Job drawing, mm, ordinate dimensions from the low corner. One solid piece. A direction names the side the tool comes from. Give positions to 0.01 mm unless a question says otherwise; leave off trailing zeros. Loops run counter-clockwise (first coordinate to the right, second up) from the corner with the lowest first, then second, coordinate; pieces in that order, holes last. Notation, with made-up numbers: (36, 48) -> (56, 48) arc R27 ccw to (56, 86) -> close; hole circle Ø9 at (7, -11). An arc over 180 degrees is marked (long way). Use one line per item in the form item = value.
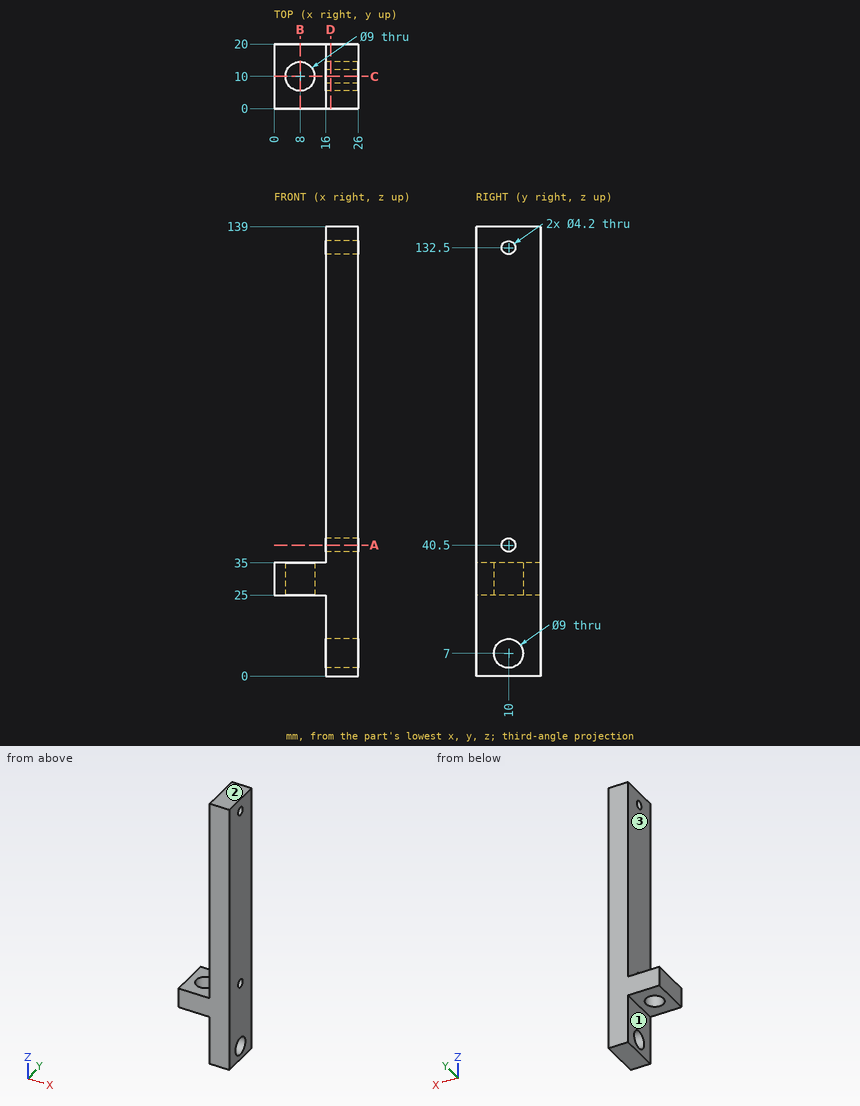
1. Cut at A-A, the plane z = 40.5. Write the cut outline in (x, y), then the cut area to 3 significant figures.
Result sheet:
outline = (16, 0) -> (26, 0) -> (26, 7.9) -> (16, 7.9) -> close; (16, 12.1) -> (26, 12.1) -> (26, 20) -> (16, 20) -> close
area = 158 mm^2
2. Cut at C-C, the plane y = 10. Write the cut outline in (x, z).
Result sheet:
outline = (0, 25) -> (3.5, 25) -> (3.5, 35) -> (0, 35) -> close; (12.5, 25) -> (16, 25) -> (16, 11.5) -> (26, 11.5) -> (26, 38.4) -> (16, 38.4) -> (16, 35) -> (12.5, 35) -> close; (16, 0) -> (26, 0) -> (26, 2.5) -> (16, 2.5) -> close; (16, 42.6) -> (26, 42.6) -> (26, 130.4) -> (16, 130.4) -> close; (16, 134.6) -> (26, 134.6) -> (26, 139) -> (16, 139) -> close
3. Cut at B-B, the plane x = 8. Write the cut outline in (y, z).
Result sheet:
outline = (0, 25) -> (5.5, 25) -> (5.5, 35) -> (0, 35) -> close; (14.5, 25) -> (20, 25) -> (20, 35) -> (14.5, 35) -> close
4. Drill centre lines: line 1 (Z direction, x = 21.25, y = 10); line 2 (Y direction, x = 22.25, z = 132.5); line 3 (Z direction, x = 20.5, y = 9.5). Where is each one in solid material? Low to high.
Result sheet:
line_1 = 0 to 2.5, 11.5 to 38.4, 42.6 to 130.4, 134.6 to 139
line_2 = 0 to 7.9, 12.1 to 20
line_3 = 0 to 2.53, 11.47 to 38.46, 42.54 to 130.46, 134.54 to 139
5. Drop flat-ended pins along their axis: P1, Ø12, axis at y = 13, z = 120, coming from the -X side; P2, Ø8, axis at x = 3, y = 16.5, coming from the -Z side. Give the stop position or say it passes through.
Result sheet:
P1 = 16
P2 = 25
6. Cut at D-D, the plane x = 17.5. Write the cut outline in (y, z).
Result sheet:
outline = (0, 0) -> (20, 0) -> (20, 139) -> (0, 139) -> close; hole circle Ø9 at (10, 7); hole circle Ø4.2 at (10, 40.5); hole circle Ø4.2 at (10, 132.5)
7. Tool access for the marked faces 1, 2 and 3: list every direction of +Z, -Z, +X, -X, +Y, -Y with a clear straight run to the whole face (end or side of a thin tool).
Result sheet:
face_1 = -Z, -X, +Y, -Y
face_2 = +Z, +X, -X, +Y, -Y
face_3 = +Z, -X, +Y, -Y
